Input: part model. Units: mm. Frame: model coordinates. Coordinates: 2 decimals unless noted, no trailing zeros. Order: outer loops, then holes, each group sorted by start corner. A loop starts at its lowest first (then second) coordinate and runs counter-clockwise, first axis right, second up. Notation, with made-up numbers: (-15, -28.75) -> (32, -28.75) arc R22 ccw to (32, -17.75) -> close; hole circle Ø11 at (39.25, 44.25). An arc over 180 degrees is marked (long way). Use one line per item in the form item = value. Start each with the question number.
1) Section query B-B on z = 41. Output: boundary loops of the cut face in (x, y).
2) Section query A-A on y = 7. Output: boundary loops of the cut face in (x, z), then the cut area to 3 significant figures.
3) Ray query, line 1 along X through (y, z) = (-19, 43.5); line 2 along X through (y, z) = (-4, 30). Return the intervals inside material, ascending.
4) Pin query (flat end, axial travel): pin 1 (1 mm diameter, centred on y = -11.5, z = 45.5, fed in from -X); pin 2 (3 mm diameter, centred on y = -14.5, z = 17.5, fed in from -X); pin 3 (3 mm diameter, centred on y = -9, z = 43.5, fed in from +X). Return the tip coordinate at first contact, or that it passes through.
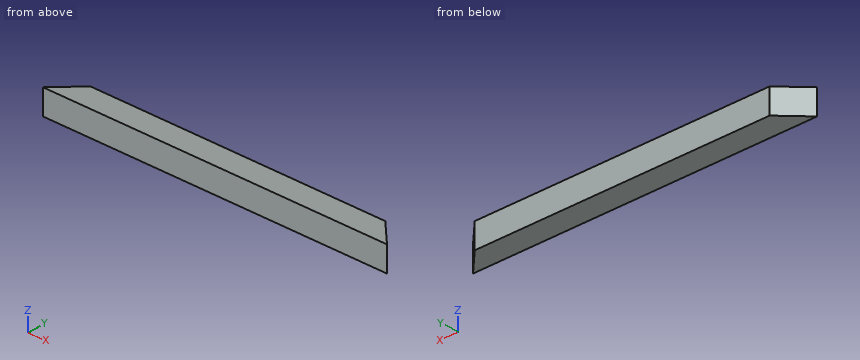
from build123d import *

# Parameters (mm, degrees)
CROQUIS1_W              = 711.2
CROQUIS1_H              = 50.8
SALIENTE_EXTRUIR1_DEPTH = 50.8
CORTAR_EXTRUIR1_DEPTH   = 361.10715072
CORTAR_EXTRUIR2_DEPTH   = 361.10715072


with BuildPart() as part:
    # Croquis1 → Saliente-Extruir1 (new body)
    with BuildSketch(Plane.XY):
        Rectangle(CROQUIS1_W, CROQUIS1_H)
    extrude(amount=SALIENTE_EXTRUIR1_DEPTH)

    # Croquis2 → Cortar-Extruir1 (cut, through all)
    with BuildSketch(Plane.XY.offset(50.8)):
        Polygon((355.6, 25.4), (335.6, 25.4), (355.6, -25.4), align=None)
        Polygon((-335.6, 25.4), (-355.6, 25.4), (-355.6, -25.4), align=None)
    extrude(amount=-CORTAR_EXTRUIR1_DEPTH, mode=Mode.SUBTRACT)

    # Croquis3 → Cortar-Extruir2 (cut, through all)
    with BuildSketch(Plane.XY.offset(50.8)):
        Polygon((-335.6, 25.4), (-355.6, -25.4), (-304.8, 25.4), align=None)
        Polygon((335.6, 25.4), (304.8, 25.4), (355.6, -25.4), align=None)
    extrude(amount=-CORTAR_EXTRUIR2_DEPTH, mode=Mode.SUBTRACT)


solid = part.part
Answers below:
q1.outline = (-355.6, -25.4) -> (355.6, -25.4) -> (304.8, 25.4) -> (-304.8, 25.4) -> close
q2.outline = (-323.2, 0) -> (323.2, 0) -> (323.2, 50.8) -> (-323.2, 50.8) -> close
q2.area = 32,800 mm^2
q3.line_1 = -349.2 to 349.2
q3.line_2 = -334.2 to 334.2
q4.pin_1 = -342.2
q4.pin_2 = -346.2
q4.pin_3 = 340.7
